Can you work these out from the model? Positions are in its coordinate system, mm. Face numbers are marked on the shaded views. Round coordinates to 2 decimals unless told otherwise and drop trailing zeros. Write each loop counter-clockwise with the first axis right and the second up, starting at its lowest first coordinate (ties: lowest second). Pieces come first, ordered by that corner, then holes.
Q1. Please list where these lines run through material, in increasing order: line 1 along Y through (x, z) = (-2.3, -19); line 2 along Z through (x, y) = (-3.95, 35); line 3 along Y through (x, z) = (-3.6, -83).
Q2. If we section it at D-D (z = -43): Please give me the cut outline in (x, y), plus the area to 3 significant figures.
Q3. If we section it at B-B (x = -1.9): Please give me the cut outline in (y, z).
Q4. I'm going to push flat-ended pins straight in: pin 1 Ø1.5 at (x, z) = (-3.5, -8) entering from +Y; pin 2 Ø2.5 at (x, z) = (-3, -76.5) entering from +Y; pin 3 Ø2.5 at (x, y) = (-1.5, 30.5) entering from -Z. Where does each tip first touch, or does it pass through?
Q5. If we section it at C-C (z = -97): Please give me the cut outline in (x, y).
Q6. We'd pull the mould along X, two halves only. Please class the marked faces 1 and 2: +X half, -X half, draft (parallel to the pull), parting line (faces both ways), or undercut.
Q7. If we section it at A-A (y = -18): Please give me the cut outline in (x, z), plus the area to 3 significant figures.
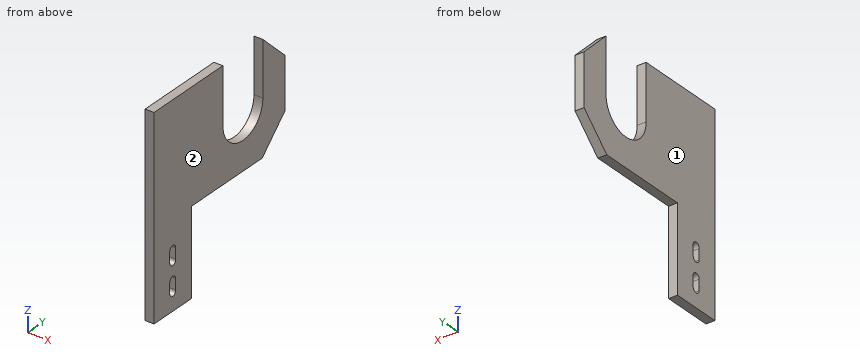
from build123d import *

# Parameters (mm, degrees)
RESSALTO_EXTRUS_O2_DEPTH = 5
RESSALTO_EXTRUS_O3_DEPTH = 5


with BuildPart() as part:
    # Esboço2 → Ressalto-extrusão2 (new body)
    with BuildSketch(Plane(origin=(0, 0, 0), x_dir=(0, 0, -1), z_dir=(1, 0, 0))):
        with BuildLine():
            Line((0.485294118, 49.5), (16.5, 66))
            Line((16.5, 66), (45.5, 66))
            Line((45.5, 66), (62, 49))
            Line((62, 49), (62, 0))
            Line((62, 0), (0, 0))
            Line((0, 0), (0, 19.5))
            Line((0, 19.5), (31, 19.5))
            ThreePointArc((31, 19.5), (46, 34.5), (31, 49.5))
            Line((31, 49.5), (0.485294118, 49.5))
        make_face()
    extrude(amount=-RESSALTO_EXTRUS_O2_DEPTH)

    # Esboço3 → Ressalto-extrusão3 (add)
    with BuildSketch(Plane(origin=(0, 0, 0), x_dir=(0, 0, -1), z_dir=(1, 0, 0))):
        Polygon((0, 0), (62, 0), (62, -4), (110, -4), (110, -32), (0, -32), align=None)
        with BuildLine():
            Line((78, -15.75), (84, -15.75))
            ThreePointArc((84, -15.75), (86.25, -18), (84, -20.25))
            Line((84, -20.25), (78, -20.25))
            ThreePointArc((78, -20.25), (75.75, -18), (78, -15.75))
        make_face(mode=Mode.SUBTRACT)
        with BuildLine():
            Line((94, -15.75), (100, -15.75))
            ThreePointArc((100, -15.75), (102.25, -18), (100, -20.25))
            Line((100, -20.25), (94, -20.25))
            ThreePointArc((94, -20.25), (91.75, -18), (94, -15.75))
        make_face(mode=Mode.SUBTRACT)
    extrude(amount=-RESSALTO_EXTRUS_O3_DEPTH)


solid = part.part
A:
1. line 1: y = -32 to 19.5, 49.5 to 66
1. line 2: z = -62 to -45.99
1. line 3: y = -32 to -20.25, -15.75 to -4
2. outline: (-5, -32) - (0, -32) - (0, 25.5) - (-5, 25.5) - close; (-5, 43.5) - (0, 43.5) - (0, 66) - (-5, 66) - close
2. area: 400 mm2
3. outline: (-32, -110) - (-4, -110) - (-4, -62) - (49, -62) - (66, -45.5) - (66, -16.5) - (49.5, -0.49) - (49.5, -31) arc R15 cw to (19.5, -31) - (19.5, 0) - (-32, 0) - close; hole (-20.25, -100) arc R2.25 ccw to (-15.75, -100) - (-15.75, -94) arc R2.25 ccw to (-20.25, -94) - close; hole (-20.25, -84) arc R2.25 ccw to (-15.75, -84) - (-15.75, -78) arc R2.25 ccw to (-20.25, -78) - close
4. pin 1: stops at y = 58.02
4. pin 2: stops at y = -4
4. pin 3: stops at z = -62
5. outline: (-5, -32) - (0, -32) - (0, -20.25) - (-5, -20.25) - close; (-5, -15.75) - (0, -15.75) - (0, -4) - (-5, -4) - close
6. face 1: -X half
6. face 2: +X half
7. outline: (-5, -110) - (0, -110) - (0, -102.25) - (-5, -102.25) - close; (-5, -91.75) - (0, -91.75) - (0, -86.25) - (-5, -86.25) - close; (-5, -75.75) - (0, -75.75) - (0, 0) - (-5, 0) - close
7. area: 445 mm2
